The model under review builds one solid part; all positions refer to its coordinate system, in mm. Face numbers are marked on the shaded views. Give positions to 0.01 mm unless a question says otherwise; leave off trailing zeros. Loops run counter-clockwise (first coordinate to the right, second up) from the corner with the lowest first, then second, coordinate; pieces in that order, holes last. Notation, with made-up numbers: (-9, 29.5) - (47, 29.5) arc R15 ccw to (47, 43.5) - close; hole circle Ø1 at (0.25, -32). An arc over 180 degrees is marked (long way). Return JSON: item names as keys, results as strings. Group by question number.
from build123d import *

# Parameters (mm, degrees)
SKETCH1_R           = 3.81
BASE_EXTRUDE_DEPTH  = 13.462
BOSS_EXTRUDE4_DEPTH = 66.167
SKETCH3_R           = 6.35
BOSS_EXTRUDE5_DEPTH = 3.048
CUT_EXTRUDE1_DEPTH  = 11.049
SKETCH5_R           = 1.3890625
CUT_EXTRUDE2_DEPTH  = 3.81


with BuildPart() as part:
    # Sketch1 → Base-Extrude (new body)
    with BuildSketch(Plane(origin=(0, 0, 0), x_dir=(0, 0, -1), z_dir=(1, 0, 0))):
        Circle(SKETCH1_R)
    extrude(amount=BASE_EXTRUDE_DEPTH)

    # Sketch2 → Boss-Extrude4 (add)
    with BuildSketch(Plane(origin=(13.462, 0, 0), x_dir=(0, 0, -1), z_dir=(1, 0, 0))):
        with BuildLine():
            Line((1.27, -3.592102448), (1.27, -1.27))
            Line((1.27, -1.27), (3.592102448, -1.27))
            ThreePointArc((3.592102448, -1.27), (3.81, 0), (3.592102448, 1.27))
            Line((3.592102448, 1.27), (1.27, 1.27))
            Line((1.27, 1.27), (1.27, 3.592102448))
            ThreePointArc((1.27, 3.592102448), (0, 3.81), (-1.27, 3.592102448))
            Line((-1.27, 3.592102448), (-1.27, 1.27))
            Line((-1.27, 1.27), (-3.592102448, 1.27))
            ThreePointArc((-3.592102448, 1.27), (-3.81, 0), (-3.592102448, -1.27))
            Line((-3.592102448, -1.27), (-1.27, -1.27))
            Line((-1.27, -1.27), (-1.27, -3.592102448))
            ThreePointArc((-1.27, -3.592102448), (0, -3.81), (1.27, -3.592102448))
        make_face()
    extrude(amount=BOSS_EXTRUDE4_DEPTH)

    # Sketch3 → Boss-Extrude5 (add)
    with BuildSketch(Plane(origin=(79.629, 0, 0), x_dir=(0, 0, -1), z_dir=(1, 0, 0))):
        with Locations(Location((0, 0, 0), (0, 0, 180))):
            Circle(SKETCH3_R)
    extrude(amount=BOSS_EXTRUDE5_DEPTH)

    # Sketch4 → Cut-Extrude1 (cut)
    with BuildSketch(Plane.ZY):
        with BuildLine():
            Line((3.463516096, 1.5875), (3.463516096, -1.5875))
            ThreePointArc((3.463516096, -1.5875), (3.81, 0), (3.463516096, 1.5875))
        make_face()
    extrude(amount=-CUT_EXTRUDE1_DEPTH, mode=Mode.SUBTRACT)

    # Sketch5 → Cut-Extrude2 (cut)
    with BuildSketch(Plane.XY.offset(3.463516096)):
        with Locations((5.08, 0)):
            Circle(SKETCH5_R)
    extrude(amount=-CUT_EXTRUDE2_DEPTH, mode=Mode.SUBTRACT)


solid = part.part
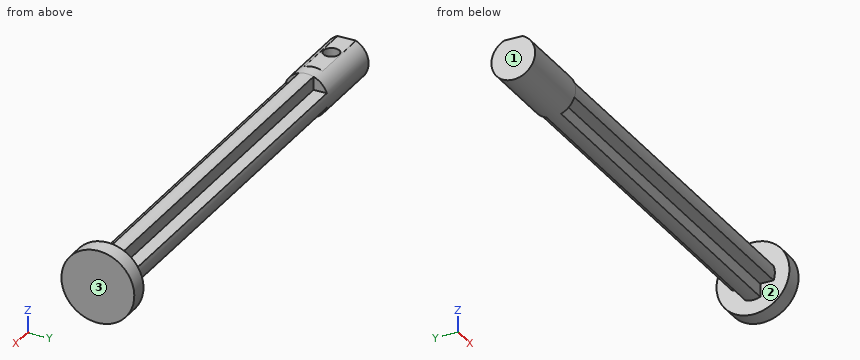
Item 1: Take a section at B-B (x = 35). State the section outline as (y, z) points.
Item 2: Mouldability with a two-part tool opening along X and no side actions: class the marked faces 1, 2 and 3 as +X half, -X half, draft (parallel to the pull), parting line (faces both ways), or undercut.
Item 3: For L1, parallel to X at y = 1.5, z = 3; L2, parallel to Z at x = 67, y = 3.5; L3, parallel to Y at x = 5.08, z = 0.95, list the stretches that pass through material, from the lowest coordinate up. Write a range as from..to.
Item 4: Take a section at A-A (y = 0). State the section outline as (x, z) points.
Item 5: Take a section at C-C (z = 2.75). State the section outline as (x, y) points.
Item 6: For P1, Ø2, axis at x = 38.5, y = 4, coming from the +Z side; P2, Ø0.8, axis at x = 5, y = -0.5, coming from the +Z side; P3, Ø1.9, axis at x = 52, z = -2.5, coming from the +Y side, all flat-tipped, find the tip position at first contact; note any pin that passes through.
Item 7: Take a section at D-D (x = 5.08). State the section outline as (y, z) points, then the cut area to 3 significant figures.
Check sheet entries:
{
 "1": {"outline": "(-3.59, -1.27) - (-1.27, -1.27) - (-1.27, -3.59) arc R3.81 ccw to (1.27, -3.59) - (1.27, -1.27) - (3.59, -1.27) arc R3.81 ccw to (3.59, 1.27) - (1.27, 1.27) - (1.27, 3.59) arc R3.81 ccw to (-1.27, 3.59) - (-1.27, 1.27) - (-3.59, 1.27) arc R3.81 ccw to start"},
 "2": {"face 1": "-X half", "face 2": "undercut", "face 3": "+X half"},
 "3": {"L1": "x = 0..13.46, 79.63..82.68", "L2": "z = -1.27..1.27", "L3": "y = -3.69..-1.39, 1.39..3.69"},
 "4": {"outline": "(0, -3.81) - (79.63, -3.81) - (79.63, -6.35) - (82.68, -6.35) - (82.68, 6.35) - (79.63, 6.35) - (79.63, 3.81) - (11.05, 3.81) - (11.05, 3.46) - (6.47, 3.46) - (6.47, -0.35) - (3.69, -0.35) - (3.69, 3.46) - (0, 3.46) - close"},
 "5": {"outline": "(0, -2.64) - (13.46, -2.64) - (13.46, -1.27) - (79.63, -1.27) - (79.63, -5.72) - (82.68, -5.72) - (82.68, 5.72) - (79.63, 5.72) - (79.63, 1.27) - (13.46, 1.27) - (13.46, 2.64) - (0, 2.64) - close; hole circle Ø2.78 at (5.08, 0)"},
 "6": {"P1": "stops at z = 1.27", "P2": "stops at z = -0.35", "P3": "stops at y = 1.27"},
 "7": {"outline": "(-1.59, 3.46) arc R3.81 ccw (long way) to (1.59, 3.46) - (1.39, 3.46) - (1.39, -0.35) - (-1.39, -0.35) - (-1.39, 3.46) - close", "area": "34.3 mm^2"}
}
